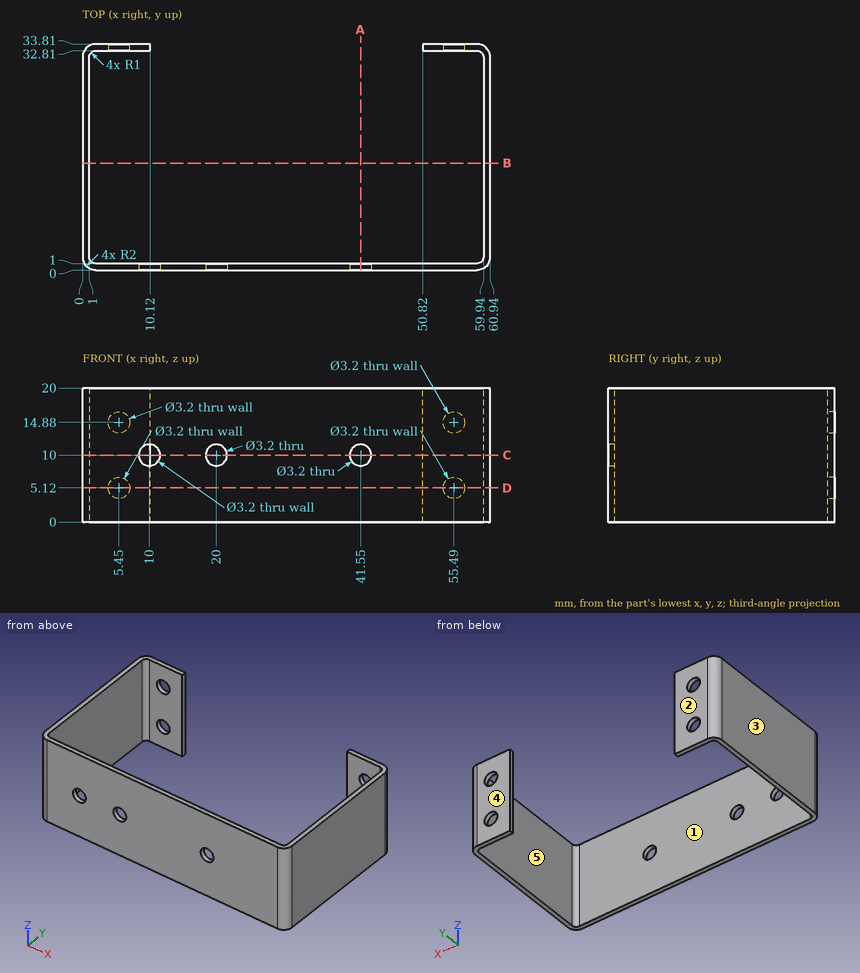
Check sheet for the drawn part. Datum: minimum x, y, z corner. Units: mm. A direction names the side the tool comes from. Coordinates: 2 decimals unless noted, no trailing zeros. Order: outer loops, then holes, each group sorted by start corner. A loop starts at its lowest first (then second) coordinate and runs counter-clockwise, first axis right, second up. Notation, with made-up numbers: (11, 65.5) -> (29, 65.5) arc R17 cw to (29, 97.5) -> close; hole circle Ø3 at (51, -7.5). An arc over 180 degrees is marked (long way). Use a Markdown table: item, result. Add a question column.
1. Set-up check for the marked faces 1 and 2: record each of +Z, -Z, +X, -X, +Y, -Y from which the full face is reachable in a straight line by a thin tool's end or side.
2. Cross-section at D-D (z = 5.12). Enter the section's corners in (x, y).
3. Cross-section at B-B (y = 16). Enter the section's corners in (x, z), and give its area (3 significant figures).
4. Cross-section at A-A (x = 41.55). Enter the section's corners in (y, z), and give its area (3 significant figures).
5. Material ranges on L1, parallel to Z at x = 55.49, y = 33.4; L2, parallel to X at y = 16.5, z = 5.5; L3, parallel to X at y = 33.5, z = 14.88, recorded low to high.
6. Cross-section at C-C (z = 10). Give the number of separate pieces and of enclosed holes in the cut face, and give its area (3 significant figures).
7. Mould release check, pull along X, two halves, no side actions. Record for the marked faces 3, 4 and 5: pulls with the +X half, pulls with the -X half, needs draft (parallel to the pull), parting line crosses it, or undercut.
8. Go/stop test with flat-tipped pins: pin 1 Ø4 at (x, z) = (20, 10) entering from +Y; pin 2 Ø2.5 at (x, z) = (10, 10) entering from -Y; pin 3 Ø0.5 at (y, z) = (33, 11.5) entering from +X. Record where each tip stops, or that it passes through.
Filled sheet:
| question | item | result |
|---|---|---|
| 1 | face 1 | +Z, -Z |
| 1 | face 2 | +Z, -Z, +X, -X, +Y |
| 2 | outline | (0, 2) arc R2 ccw to (2, 0) -> (58.94, 0) arc R2 ccw to (60.94, 2) -> (60.94, 31.81) arc R2 ccw to (58.94, 33.81) -> (57.09, 33.81) -> (57.09, 32.81) -> (58.94, 32.81) arc R1 cw to (59.94, 31.81) -> (59.94, 2) arc R1 cw to (58.94, 1) -> (2, 1) arc R1 cw to (1, 2) -> (1, 31.81) arc R1 cw to (2, 32.81) -> (3.85, 32.81) -> (3.85, 33.81) -> (2, 33.81) arc R2 ccw to (0, 31.81) -> close; (7.05, 32.81) -> (10.12, 32.81) -> (10.12, 33.81) -> (7.05, 33.81) -> close; (50.82, 32.81) -> (53.89, 32.81) -> (53.89, 33.81) -> (50.82, 33.81) -> close |
| 3 | outline | (0, 0) -> (1, 0) -> (1, 20) -> (0, 20) -> close; (59.94, 0) -> (60.94, 0) -> (60.94, 20) -> (59.94, 20) -> close |
| 3 | area | 40.0 mm2 |
| 4 | outline | (0, 0) -> (1, 0) -> (1, 8.4) -> (0, 8.4) -> close; (0, 11.6) -> (1, 11.6) -> (1, 20) -> (0, 20) -> close |
| 4 | area | 16.8 mm2 |
| 5 | L1 | 0 to 3.52, 6.72 to 13.28, 16.48 to 20 |
| 5 | L2 | 0 to 1, 59.94 to 60.94 |
| 5 | L3 | 0.93 to 3.85, 7.05 to 10.12, 50.82 to 53.89, 57.09 to 60.01 |
| 6 | separate pieces | 4 |
| 6 | enclosed holes | 0 |
| 6 | area | 133 mm2 |
| 7 | face 3 | pulls with the -X half |
| 7 | face 4 | needs draft |
| 7 | face 5 | undercut |
| 8 | pin 1 | y = 1 |
| 8 | pin 2 | y = 32.81 |
| 8 | pin 3 | x = 60.71 |
